Here's how the part is built. I have some questions about the finished solid (model axes, mm). A direction names the side the tool comes from. Round coordinates to 2 decimals unless told otherwise and drop trailing zeros. Order: outer loops, then holes, each group sorted by start corner. A loop starts at its lowest first (then second) coordinate and runs counter-clockwise, first axis right, second up.
Autodesk Inventor part; units mm, degrees
ref_plane "YZ Plane" through (0, 0, 0) normal (1, 0, 0) x (0, 1, 0)
ref_plane "XZ Plane" through (0, 0, 0) normal (0, 1, 0) x (-1, 0, 0)
ref_plane "XY Plane" through (0, 0, 0) normal (0, 0, 1) x (1, 0, 0)
sketch "Sketch1" plane through (0, 0, 0) normal (0, 0, 1) x (1, 0, 0)
  line L0 (-125, 120) -> (125, 120)
  line L1 (125, 120) -> (125, -120)
  line L2 (125, -120) -> (-125, -120)
  line L3 (-125, -120) -> (-125, 120)
  point P0 (0, 0)
  dimension "d0" = 250
  dimension "d1" = 240
  dimension "d2" = 125
  dimension "d3" = 120
extrude "Extrusion1" add sketch "Sketch1" along normal mid plane 10
sketch "Sketch5" plane through (0, 0, 5) normal (0, 0, 1) x (1, 0, 0)
  line L0 (-115, 100) -> (-115, -103.2)
  line L1 (-92.14, 100) -> (-92.14, -103.2)
  line L2 (39.94, 100) -> (39.94, -103.2)
  line L3 (112.33, 100) -> (112.33, -103.2)
  line L4 (-92.14, 100) -> (112.33, 100)
  line L5 (-115, -57.48) -> (39.94, -57.48)
  line L6 (112.33, -57.48) -> (39.94, -57.48)
  line L7 (-115, -103.2) -> (39.94, -103.2)
  line L8 (112.33, -103.2) -> (39.94, -103.2)
  line L9 (-115, 100) -> (-92.14, 100)
  line L10 (-125, 120) -> (-125, -120)
  line L11 (125, 120) -> (-125, 120)
  point P0 (0, 0)
  dimension "d25" = 10
  dimension "d26" = 22.86
  dimension "d27" = 72.39
  dimension "d28" = 132.08
  dimension "d29" = 45.72
  dimension "d30" = 157.48
  dimension "d38" = 20
hole "Hole2" at (-92.14, 100, 5) at (39.94, 100, 5) at (112.33, 100, 5) at (112.33, -57.48, 5) at (39.94, -57.48, 5) at (39.94, -103.2, 5) at (112.33, -103.2, 5) at (-115, -57.48, 5) at (-115, -103.2, 5) direction (0, 0, -1) diameter 3.6 depth 5 tip angle 118
thicken "Thicken1" operation add thickness 5 both sides no extend neighbours yes toward (-1, 0, 0) faces at (-125, 40, -1.6667)
sketch "Sketch11" plane through (0, 0, 5) normal (0, 0, 1) x (1, 0, 0)
  line L0 (125, 120) -> (-130, 120)
  line L1 (-130, -120) -> (125, -120)
  line L2 (-130, 120) -> (-125, 120)
  line L3 (-125, 120) -> (-125, -120)
  line L4 (-125, -120) -> (-130, -120)
  line L5 (-130, -120) -> (-130, 120)
  point P0 (0, 0)
  dimension "d70" = 5
extrude "Extrusion5" add sketch "Sketch11" along normal blind 55
sketch "Sketch12" plane through (-130, -120, -5) normal (-1, 0, 0) x (0, 0, 1)
  line L0 (10, 221.8) -> (10, 218.2)
  line L1 (10, 220) -> (65, 220)
  line L2 (65, 240) -> (65, 0)
  line L3 (62.32, 226.75) -> (17.62, 226.75)
  line L4 (17.62, 226.75) -> (17.62, 67.75)
  line L5 (17.62, 67.75) -> (62.32, 67.75)
  line L6 (62.32, 67.75) -> (62.32, 226.75)
  line L7 (10, 240) -> (10, 0)
  line L8 (10, 0) -> (10, 240)
  line L9 (65, 0) -> (65, 240)
  line L10 (10, 54.5) -> (65, 54.5)
  line L11 (65, 54.5) -> (65, 0)
  line L12 (65, 0) -> (10, 0)
  line L13 (10, 0) -> (10, 54.5)
  point P0 (10, 0)
  point P1 (65, 54.5)
  point P2 (10, 54.5)
  dimension "d75" = 44.7
  dimension "d76" = 159
  dimension "d77" = 6.75
  dimension "d78" = 7.62
  dimension "d79" = 13.25
extrude "Extrusion6" cut sketch "Sketch12" against normal up to surface (5 mm away) contours L4 L3 L6 L1 | L1 L6 L5 L4 | L10 L2 L12 L7
ref_plane "Work Plane1" through (0, 0, -1.42) normal (0, 0, 1) x (1, 0, 0)
sketch "Sketch13" plane through (0, 0, -1.42) normal (0, 0, 1) x (1, 0, 0)
  line L0 (-130, -120) -> (-130, -65.5)
  line L1 (-130, -65.5) -> (-145, -65.5)
  line L2 (-145, -65.5) -> (-145, -120)
  line L3 (-145, -120) -> (-130, -120)
  line L4 (-130, -120) -> (-130, -65.5)
  point P0 (0, 0)
  dimension "d83" = 15
  dimension "d86" = 54.5
extrude "Extrusion7" add sketch "Sketch13" along normal blind 5
sketch "Sketch14" plane through (0, 0, 3.58) normal (0, 0, 1) x (1, 0, 0)
  line L0 (-145, -120) -> (-130, -120)
  line L1 (-131.22, -72.75) -> (-136.22, -72.75)
  line L2 (-136.22, -72.75) -> (-136.22, -112.75)
  line L3 (-136.22, -112.75) -> (-131.22, -112.75)
  line L4 (-131.22, -112.75) -> (-131.22, -72.75)
  line L5 (-130, -120) -> (-130, -65.5)
  line L6 (-125, 120) -> (-125, -65.5)
  circle A0 centre (-133.72, -72.75) radius 2.5
  circle A1 centre (-133.72, -112.75) radius 2.5
  point P0 (0, 0)
  point P1 (-137.2605, -92.75)
  dimension "d87" = 27.25
  dimension "d88" = 5
  dimension "d89" = 40
  dimension "d90" = 20
  dimension "d92" = 6.22
extrude "Extrusion8" cut sketch "Sketch14" against normal up to surface (5 mm away)
sketch "Sketch15" plane through (0, 0, 5) normal (0, 0, 1) x (1, 0, 0)
  line L0 (-125, 120) -> (-125, -65.5)
  line L1 (-145, -120) -> (-130, -120)
  line L2 (-125, -65.5) -> (-130, -65.5)
  line L3 (-130, -65.5) -> (-130, -120)
  line L4 (-130, -120) -> (-125, -120)
  line L5 (-125, -120) -> (-125, -65.5)
  point P0 (0, 0)
extrude "Extrusion9" cut sketch "Sketch15" against normal blind 1.42
thicken "Thicken2" operation add thickness 25 both sides no extend neighbours yes toward (1, 0, 0) faces at (125, -40, -1.6667)
sketch "Sketch18" plane through (0, 0, 5) normal (0, 0, 1) x (1, 0, 0)
  line L0 (150, 120) -> (-125, 120)
  line L1 (140, 105) -> (125, 105)
  line L2 (125, 105) -> (125, -105)
  line L3 (125, -105) -> (140, -105)
  line L4 (140, -105) -> (140, 105)
  line L5 (150, -120) -> (150, 120)
  line L6 (20.8941, 78.5076) -> (-64.1059, 78.5076)
  line L7 (-64.1059, 78.5076) -> (-64.1059, -6.4924)
  line L8 (-64.1059, -6.4924) -> (20.8941, -6.4924)
  line L9 (20.8941, -6.4924) -> (20.8941, 78.5076)
  point P0 (0, 0)
  point P1 (139.9053, 0)
  dimension "d102" = 120
  dimension "d103" = 15
  dimension "d104" = 210
  dimension "d105" = 105
  dimension "d106" = 10
  dimension "d107" = 85
  dimension "d108" = 85
extrude "Extrusion11" cut sketch "Sketch18" against normal up to surface (10 mm away)
chamfer "Chamfer4" distance 10 angle 45 4 edges at (-64.1059, 78.5076, 0) (-64.1059, -6.4924, 0) (20.8941, -6.4924, 0) (20.8941, 78.5076, 0)
properties part number "_3DPrint"
1. I need wall thicknesses on probe 1 along X at (y, z) = (-57.48, 3); probe 2 along X at (y, z) = (100, 1.7); probe 3 along Y at (x, z) = (39.94, 2). Which ranges of each line are inside material? Lowest first, please.
Evaluation:
probe 1: x = -130 to -116.8, -113.2 to 38.14, 41.74 to 110.53, 114.13 to 125, 140 to 150
probe 2: x = -130 to -93.94, -90.34 to 38.14, 41.74 to 110.53, 114.13 to 125, 140 to 150
probe 3: y = -120 to -105, -101.4 to -59.28, -55.68 to 98.2, 101.8 to 120
2. If we section it at C-C, the plane z = 53: Write out the boundary of the cut face in (x, y).
Evaluation:
outline: (-130, -65.5) - (-125, -65.5) - (-125, -52.25) - (-130, -52.25) - close; (-130, 106.75) - (-125, 106.75) - (-125, 120) - (-130, 120) - close
3. On a 3-axis mill with a long thin cutter (end or side, diameter ignored), from which of +Z, -Z, +X, -X, +Y, -Y can I reach the whole of each face in a straight line? I mean faces 1 (the flat face through (-139, -92, -1.42)), 2 (the flat face through (-125, 28, 8)), 3 (the flat face through (125, 1, 0)), 4 (the flat face through (-137, -92, 3.58)). Say none if no direction works.
Evaluation:
face 1: -Z, -X, +Y, -Y
face 2: +Z, +X, +Y, -Y
face 3: +Z, -Z
face 4: +Z, -X, -Y
4. I'm going to push flat-ended pins straight in: P1, Ø1.5, axis at x = -126.5, z = 35.5, coming from the -Y side; P2, Ø3, axis at x = 39.94, y = -103.2, coming from the +Z side; P3, Ø6, axis at x = -136.5, y = -95.5, coming from the +Z side. Where does each tip first touch, or does it pass through?
Evaluation:
P1: stops at y = -65.5
P2: stops at z = -0.18
P3: stops at z = 3.58
5. If we section it at B-B, the plane y = -97.5: Write out the boundary of the cut face in (x, z).
Evaluation:
outline: (-145, -1.42) - (-136.22, -1.42) - (-136.22, 3.58) - (-145, 3.58) - close; (-131.22, -1.42) - (-130, -1.42) - (-130, -5) - (125, -5) - (125, 5) - (-125, 5) - (-125, 3.58) - (-131.22, 3.58) - close; (140, -5) - (150, -5) - (150, 5) - (140, 5) - close
6. If we mould it in two halves opening along X, with no side actions, what happens to faces 5 (the flat face through (-22, -6.492, 0)), 6 (the flat face through (11, -25, 5)), 7 (the flat face through (150, 2, 0))? For each: released by +X, released by -X, zero draft, split by the parting line, or undercut.
Evaluation:
face 5: undercut
face 6: zero draft
face 7: released by +X
7. If we section it at A-A, the plane x = -3.5: Write out the boundary of the cut face in (y, z).
Evaluation:
outline: (-120, -5) - (-6.49, -5) - (-6.49, 5) - (-120, 5) - close; (78.51, -5) - (120, -5) - (120, 5) - (78.51, 5) - close
8. If we section it at D-D, the plane y = 15: Write out the boundary of the cut face in (x, z).
Evaluation:
outline: (-130, -5) - (-64.11, -5) - (-64.11, 5) - (-125, 5) - (-125, 12.62) - (-130, 12.62) - close; (-130, 57.32) - (-125, 57.32) - (-125, 60) - (-130, 60) - close; (20.89, -5) - (125, -5) - (125, 5) - (20.89, 5) - close; (140, -5) - (150, -5) - (150, 5) - (140, 5) - close
